```python
from build123d import *

# Parameters (mm, degrees)
SKETCH1_W             = 20
SKETCH1_H             = 197.5
SKETCH1_H_2           = 15
SKETCH1_W_2           = 14.875
BOSS_EXTRUDE1_DEPTH   = 10
IZIM1_W               = 10
IZIM1_H               = 130
KES_EKSTR_ZYON1_DEPTH = 15


with BuildPart() as part:
    # Sketch1 → Boss-Extrude1 (new body)
    with BuildSketch(Plane.XY):
        with Locations((0, -121.25)):
            Rectangle(SKETCH1_W, SKETCH1_H)
        with Locations((0, -15)):
            Rectangle(SKETCH1_W, SKETCH1_H_2)
        Polygon((-10, 7.5), (-10, -7.5), (10, -7.5), (10, 7.5), (5.773502692, 7.5), (2.886751346, 2.5), (-2.886751346, 2.5), (-5.773502692, 7.5), align=None)
        with Locations((-17.4375, 0)):
            Rectangle(SKETCH1_W_2, SKETCH1_H_2)
        with Locations((17.4375, 0)):
            Rectangle(SKETCH1_W_2, SKETCH1_H_2)
    extrude(amount=BOSS_EXTRUDE1_DEPTH)

    # Çizim1 → Kes-Ekstrüzyon1 (cut)
    with BuildSketch(Plane(origin=(10, 0, 0), x_dir=(0, 0, -1), z_dir=(1, 0, 0))):
        with Locations((-5, -155)):
            Rectangle(IZIM1_W, IZIM1_H)
    extrude(amount=-KES_EKSTR_ZYON1_DEPTH, mode=Mode.SUBTRACT)


solid = part.part
```
Here's how the part is built. I have some questions about the finished solid (model axes, mm). A direction names the side the tool comes from. Coordinates: 2 decimals unless noted, no trailing zeros. Order: outer loops, then holes, each group sorted by start corner. A loop starts at its lowest first (then second) coordinate and runs counter-clockwise, first axis right, second up.
Item 1: If we section it at C-C, the plane x = -21: List the corners of the cut face in (y, z) for me, then the cut area to 3 significant figures.
Response values:
outline: (-7.5, 0) - (7.5, 0) - (7.5, 10) - (-7.5, 10) - close
area: 150 mm2
Item 2: I need wall thicknesses on probe 1 along Y at (x, z) = (-13, 3.75); probe 2 along Y at (x, z) = (-0.5, 5.5); probe 3 along X at (y, z) = (-22, 6). Which ranges of each line are inside material? Lowest first, please.
Response values:
probe 1: y = -7.5 to 7.5
probe 2: y = -90 to 2.5
probe 3: x = -10 to 10
Item 3: If we section it at A-A, the plane z = 7: List the corners of the cut face in (x, y) for me (1 decimal), then the cut area to 3 significant figures.
Response values:
outline: (-24.9, -7.5) - (-10, -7.5) - (-10, -220) - (-5, -220) - (-5, -90) - (10, -90) - (10, -7.5) - (24.9, -7.5) - (24.9, 7.5) - (5.8, 7.5) - (2.9, 2.5) - (-2.9, 2.5) - (-5.8, 7.5) - (-24.9, 7.5) - close
area: 3,000 mm2
Item 4: I'm going to push flat-ended pins straight in: pin 1 Ø5 at (x, z) = (18, 2.5) entering from -Y; pin 2 Ø3 at (x, z) = (1, 6) entering from +Y; pin 3 Ø5 at (y, z) = (-141, 4.5) entering from -X. Where does each tip first touch, or does it pass through?
Response values:
pin 1: stops at y = -7.5
pin 2: stops at y = 2.5
pin 3: stops at x = -10
Item 5: If we section it at B-B, the plane y = -195: List the corners of the cut face in (x, z) for me.
Response values:
outline: (-10, 0) - (-5, 0) - (-5, 10) - (-10, 10) - close
Item 6: Thinking about a two-plate mould opening in X: for faces 4 (the face through (-10, -112, 5)), 5 (the face through (0, 2.5, 5)), 6 (the face through (3, -90, 5)), which applies, pulls with the +X half, pulls with the -X half, needs draft (parallel to the pull), parting line crosses it, or undercut?
Response values:
face 4: pulls with the -X half
face 5: undercut
face 6: needs draft
Item 7: Which directions (+Z, -Z, +X, -X, +Y, -Y) give clear straight access to the entire face, cutting with the end or side of a thin tool? Please do faces 1 (the face through (10, -49, 5)), 2 (the face through (-18, -7.5, 5)), 3 (the face through (4.35, 5.035, 4.93)).
Response values:
face 1: +Z, -Z, +X, -Y
face 2: +Z, -Z, -X, -Y
face 3: +Z, -Z, +Y
